Part model, mm, in its own coordinate system. Face numbers are marked on the shaded views. Coordinates: 2 decimals unless noted, no trailing zeros. Write each loop counter-clockwise with the first axis right and the second up, starting at its lowest first coordinate (ties: lowest second). Pieces come first, ordered by that corner, then holes. Notation, with made-up numbers: M 80.5,-40 L 104.5,-40 A21 ccw 104.5,-19 Z; hole C -31,23.5 d8. An arc over 180 degrees is marked long. Use a Markdown table: item, result. Add a question column.
Q1. Slice it at B-B on x = -35. Write the cut outline in (y, z), then the cut area to 3 significant figures.
Q2. Slice it at A-A on y = -41. Write the cut outline in (x, z), then the cut area to 3 significant figures.
Q3. Pin check, flat tips, straight feed: pin 1 Ø0.5 at (y, z) = (-13, 0.5) entering from -X; pin 2 Ø2 at (x, y) = (-32.5, -24.9) entering from -Z. Stop position of each tip, or through.
Q4. Wall check: L1, parallel to Y at x = 34.5, z = 0.7; L2, parallel to X at y = 1, z = 1.15; L3, parallel to Z at x = -26, y = -34. Give the ranges that are in metal, low to high. Write a range as from..to.
Q5. Slice it at C-C on y = 3. Write the cut outline in (x, z), then the cut area to 3 significant figures.
Q6. Slice it at D-D on x = -6. Write the cut outline in (y, z), then the cut area to 3 significant figures.
Q7. Mould opens along X. For the marked faces 1 and 2 say: released by +X, released by -X, zero draft, split by the parting line, or undercut.
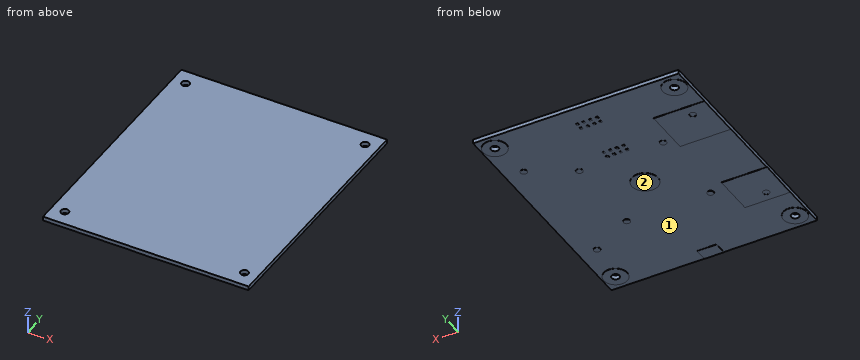
from build123d import *

# Parameters (mm, degrees)
SKETCH1_W           = 79
SKETCH1_H           = 94
SKETCH1_R           = 1.5
BOSS_EXTRUDE1_DEPTH = 1.6
BOSS_EXTRUDE2_START = -0.1
SKETCH2_R           = 5
SKETCH2_R_2         = 1.25
SKETCH2_R_3         = 4.5
SKETCH2_R_4         = 1.5
SKETCH2_W           = 0.889
SKETCH2_H           = 0.889
SKETCH2_W_2         = 19.5
SKETCH2_H_2         = 18
SKETCH2_W_3         = 7.5
SKETCH2_H_3         = 4.995279521
BOSS_EXTRUDE2_DEPTH = 0.1


with BuildPart() as part:
    # Sketch1 → Boss-Extrude1 (new body)
    with BuildSketch(Plane.XY):
        Rectangle(SKETCH1_W, SKETCH1_H)
        with Locations((-34.5, 41)):
            Circle(SKETCH1_R, mode=Mode.SUBTRACT)
        with Locations(Location((34.5, 41, 0), (0, 0, 180))):
            Circle(SKETCH1_R, mode=Mode.SUBTRACT)
        with Locations((34.5, -41)):
            Circle(SKETCH1_R, mode=Mode.SUBTRACT)
        with Locations(Location((-34.5, -41, 0), (0, 0, 180))):
            Circle(SKETCH1_R, mode=Mode.SUBTRACT)
    extrude(amount=BOSS_EXTRUDE1_DEPTH)

    # Sketch2 → Boss-Extrude2 (add)
    # profile 1 of 30: a face of its own
    with BuildSketch(Plane.XY.offset(BOSS_EXTRUDE2_START)):
        Circle(SKETCH2_R)
    # profile 2 of 30: a face of its own
    with BuildSketch(Plane.XY.offset(BOSS_EXTRUDE2_START)):
        with Locations((-16.086679272, 16.086679272)):
            Circle(SKETCH2_R_2)
    # profile 3 of 30: a face of its own
    with BuildSketch(Plane.XY.offset(BOSS_EXTRUDE2_START)):
        with Locations((16.086679272, 16.086679272)):
            Circle(SKETCH2_R_2)
    # profile 4 of 30: a face of its own
    with BuildSketch(Plane.XY.offset(BOSS_EXTRUDE2_START)):
        with Locations((32.5, 24.9)):
            Circle(SKETCH2_R_2)
    # profile 5 of 30: a face of its own
    with BuildSketch(Plane.XY.offset(BOSS_EXTRUDE2_START)):
        with Locations((16.086679272, -16.086679272)):
            Circle(SKETCH2_R_2)
    # profile 6 of 30: a face of its own
    with BuildSketch(Plane.XY.offset(BOSS_EXTRUDE2_START)):
        with Locations((32.5, -24.9)):
            Circle(SKETCH2_R_2)
    # profile 7 of 30: a face of its own
    with BuildSketch(Plane.XY.offset(BOSS_EXTRUDE2_START)):
        with Locations((-16.086679272, -16.086679272)):
            Circle(SKETCH2_R_2)
    # profile 8 of 30: a face of its own
    with BuildSketch(Plane.XY.offset(BOSS_EXTRUDE2_START)):
        with Locations((-34.5, 41)):
            Circle(SKETCH2_R_3)
        with Locations((-34.5, 41)):
            Circle(SKETCH2_R_4, mode=Mode.SUBTRACT)
    # profile 9 of 30: a face of its own
    with BuildSketch(Plane.XY.offset(BOSS_EXTRUDE2_START)):
        with Locations(Location((34.5, 41, 0), (0, 0, 180))):
            Circle(SKETCH2_R_3)
        with Locations(Location((34.5, 41, 0), (0, 0, 180))):
            Circle(SKETCH2_R_4, mode=Mode.SUBTRACT)
    # profile 10 of 30: a face of its own
    with BuildSketch(Plane.XY.offset(BOSS_EXTRUDE2_START)):
        with Locations(Location((-34.5, -41, 0), (0, 0, 180))):
            Circle(SKETCH2_R_3)
        with Locations(Location((-34.5, -41, 0), (0, 0, 180))):
            Circle(SKETCH2_R_4, mode=Mode.SUBTRACT)
    # profile 11 of 30: a face of its own
    with BuildSketch(Plane.XY.offset(BOSS_EXTRUDE2_START)):
        with Locations((34.5, -41)):
            Circle(SKETCH2_R_3)
        with Locations((34.5, -41)):
            Circle(SKETCH2_R_4, mode=Mode.SUBTRACT)
    # profile 12 of 30: a face of its own
    with BuildSketch(Plane.XY.offset(BOSS_EXTRUDE2_START)):
        with Locations((-3.72, 39.1133)):
            Rectangle(SKETCH2_W, SKETCH2_H)
    # profile 13 of 30: a face of its own
    with BuildSketch(Plane.XY.offset(BOSS_EXTRUDE2_START)):
        with Locations((-1.18, 39.1133)):
            Rectangle(SKETCH2_W, SKETCH2_H)
    # profile 14 of 30: a face of its own
    with BuildSketch(Plane.XY.offset(BOSS_EXTRUDE2_START)):
        with Locations((1.36, 39.1133)):
            Rectangle(SKETCH2_W, SKETCH2_H)
    # profile 15 of 30: a face of its own
    with BuildSketch(Plane.XY.offset(BOSS_EXTRUDE2_START)):
        with Locations((3.9, 39.1133)):
            Rectangle(SKETCH2_W, SKETCH2_H)
    # profile 16 of 30: a face of its own
    with BuildSketch(Plane.XY.offset(BOSS_EXTRUDE2_START)):
        with Locations((-3.72, 36.5733)):
            Rectangle(SKETCH2_W, SKETCH2_H)
    # profile 17 of 30: a face of its own
    with BuildSketch(Plane.XY.offset(BOSS_EXTRUDE2_START)):
        with Locations((-1.18, 36.5733)):
            Rectangle(SKETCH2_W, SKETCH2_H)
    # profile 18 of 30: a face of its own
    with BuildSketch(Plane.XY.offset(BOSS_EXTRUDE2_START)):
        with Locations((1.36, 36.5733)):
            Rectangle(SKETCH2_W, SKETCH2_H)
    # profile 19 of 30: a face of its own
    with BuildSketch(Plane.XY.offset(BOSS_EXTRUDE2_START)):
        with Locations((3.9, 36.5733)):
            Rectangle(SKETCH2_W, SKETCH2_H)
    # profile 20 of 30: a face of its own
    with BuildSketch(Plane.XY.offset(BOSS_EXTRUDE2_START)):
        with Locations((-3.72, 21.1133)):
            Rectangle(SKETCH2_W, SKETCH2_H)
    # profile 21 of 30: a face of its own
    with BuildSketch(Plane.XY.offset(BOSS_EXTRUDE2_START)):
        with Locations((-1.18, 21.1133)):
            Rectangle(SKETCH2_W, SKETCH2_H)
    # profile 22 of 30: a face of its own
    with BuildSketch(Plane.XY.offset(BOSS_EXTRUDE2_START)):
        with Locations((1.36, 21.1133)):
            Rectangle(SKETCH2_W, SKETCH2_H)
    # profile 23 of 30: a face of its own
    with BuildSketch(Plane.XY.offset(BOSS_EXTRUDE2_START)):
        with Locations((3.9, 21.1133)):
            Rectangle(SKETCH2_W, SKETCH2_H)
    # profile 24 of 30: a face of its own
    with BuildSketch(Plane.XY.offset(BOSS_EXTRUDE2_START)):
        with Locations((-3.72, 18.5733)):
            Rectangle(SKETCH2_W, SKETCH2_H)
    # profile 25 of 30: a face of its own
    with BuildSketch(Plane.XY.offset(BOSS_EXTRUDE2_START)):
        with Locations((-1.18, 18.5733)):
            Rectangle(SKETCH2_W, SKETCH2_H)
    # profile 26 of 30: a face of its own
    with BuildSketch(Plane.XY.offset(BOSS_EXTRUDE2_START)):
        with Locations((1.36, 18.5733)):
            Rectangle(SKETCH2_W, SKETCH2_H)
    # profile 27 of 30: a face of its own
    with BuildSketch(Plane.XY.offset(BOSS_EXTRUDE2_START)):
        with Locations((3.9, 18.5733)):
            Rectangle(SKETCH2_W, SKETCH2_H)
    # profile 28 of 30: a face of its own
    with BuildSketch(Plane.XY.offset(BOSS_EXTRUDE2_START)):
        with Locations((-29.75, 20.5)):
            Rectangle(SKETCH2_W_2, SKETCH2_H_2)
        with Locations((-32.5, 24.9)):
            Circle(SKETCH2_R_2, mode=Mode.SUBTRACT)
    # profile 29 of 30: a face of its own
    with BuildSketch(Plane.XY.offset(BOSS_EXTRUDE2_START)):
        with Locations((0, -44.502360239)):
            Rectangle(SKETCH2_W_3, SKETCH2_H_3)
    # profile 30 of 30: a face of its own
    with BuildSketch(Plane.XY.offset(BOSS_EXTRUDE2_START)):
        Polygon((-39.724379768, -12.8), (-22.135781761, -12.8), (-22.135781761, -28.8), (-39.499973122, -28.8), align=None)
        with Locations((-32.5, -24.9)):
            Circle(SKETCH2_R_2, mode=Mode.SUBTRACT)
    extrude(amount=BOSS_EXTRUDE2_DEPTH)


solid = part.part
Recorded:
| question | item | result |
|---|---|---|
| 1 | outline | M -47,0 L -45.47,0 L -45.47,-0.1 L -42.41,-0.1 L -42.41,1.6 L -47,1.6 Z; M -39.59,-0.1 L -36.53,-0.1 L -36.53,0 L -28.8,0 L -28.8,-0.1 L -12.8,-0.1 L -12.8,0 L 11.5,0 L 11.5,-0.1 L 29.5,-0.1 L 29.5,0 L 36.53,0 L 36.53,-0.1 L 39.59,-0.1 L 39.59,1.6 L -39.59,1.6 Z; M 42.41,-0.1 L 45.47,-0.1 L 45.47,0 L 47,0 L 47,1.6 L 42.41,1.6 Z |
| 1 | area | 146 mm² |
| 2 | outline | M -39.5,0 L -39,0 L -39,-0.1 L -36,-0.1 L -36,1.6 L -39.5,1.6 Z; M -33,-0.1 L -30,-0.1 L -30,0 L 30,0 L 30,-0.1 L 33,-0.1 L 33,1.6 L -33,1.6 Z; M 36,-0.1 L 39,-0.1 L 39,0 L 39.5,0 L 39.5,1.6 L 36,1.6 Z |
| 2 | area | 118 mm² |
| 3 | pin 1 | x = -39.5 |
| 3 | pin 2 | z = 0 |
| 4 | L1 | -47..-42.5, -39.5..39.5, 42.5..47 |
| 4 | L2 | -39.5..39.5 |
| 4 | L3 | 0..1.6 |
| 5 | outline | M -39.5,0 L -4,0 L -4,-0.1 L 4,-0.1 L 4,0 L 39.5,0 L 39.5,1.6 L -39.5,1.6 Z |
| 5 | area | 127 mm² |
| 6 | outline | M -47,0 L 47,0 L 47,1.6 L -47,1.6 Z |
| 6 | area | 150 mm² |
| 7 | face 1 | undercut |
| 7 | face 2 | zero draft |
